Model file for the job. Use its own axes, mm. Face numbers are marked on the shaded views. A direction names the side the tool comes from. Coordinates: 2 decimals unless noted, no trailing zeros. Write each loop counter-clockwise with the first axis right and the second up, starting at its lowest first coordinate (ties: lowest second). Pieces come first, ordered by that corner, then holes. Notation, with made-up numbers: M 32.5,14.25 L 67.5,14.25 A6 ccw 67.5,22.25 Z; hole C -22.75,75 d6. An arc over 180 degrees is marked long. One line per question, with ' | ' between items. Start each with the question number.
(1) Two-plate mould, pull along X, no slides. Class the marked faces 3, 4 and 5: +X half, -X half, draft (parallel to the pull), parting line (faces both ways), or undercut.
(2) Tool access for the marked faces 1 and 2: list every direction of +Z, -Z, +X, -X, +Y, -Y with a clear straight run to the whole face (end or side of a thin tool).
(3) Flat gauge pins, fed straight in: pin 1 Ø2 at (x, y) = (-4, 3.5) entering from -Z; pin 2 Ø6.5 at (x, y) = (0, 0) entering from +Z; pin 3 Ø1.5 at (y, z) = (-3.5, 1.5) entering from +X. Where does each tip first touch, or does it go through?
(4) Wall check: probe 1 along Y at (x, z) = (0, 1.2); probe 2 along Z at (x, y) = (-6, -2); probe 3 along Z at (x, y) = (-2, 1.75). Give the ranges that are in metal, low to high.
(5) Cut at C-C (y = 0). Write the cut outline in (x, z).
(6) Cut at B-B (z = 1.2). Write the cut outline in (x, y), plus the area to 3 significant figures.
(7) Cut at A-A (x = 0). Write the cut outline in (y, z), plus the area to 3 significant figures.
from build123d import *

# Parameters (mm, degrees)
SKETCH_R        = 2.5
PAD_DEPTH       = 0.6
SKETCH002_R     = 9.5
PAD001_DEPTH    = 1
SKETCH003_R     = 9.5
SKETCH003_R_2   = 8
PAD002_DEPTH    = 1
SKETCH004_R     = 2.5
POCKET_DEPTH    = 1.601
CHAMFER_SIZE    = 0.4
CHAMFER001_SIZE = 0.2


with BuildPart() as part:
    # Sketch → Pad (new body)
    with BuildSketch(Plane.XY):
        with BuildLine():
            ThreePointArc((-2.5, 3.122499), (-3.518971, 1.901799), (-3.981855, 0.380567))
            Line((-5.478695, -0.483634), (-3.981855, 0.380567))
            ThreePointArc((-5.478695, -0.483634), (-4.659167, -2.922699), (-2.81991, -4.722087))
            Line((-1.232265, -3.80546), (-2.81991, -4.722087))
            ThreePointArc((-1.232265, -3.80546), (0.117848, -3.998264), (1.454262, -3.726275))
            Line((2.992718, -4.614503), (1.454262, -3.726275))
            ThreePointArc((2.992718, -4.614503), (4.763149, -2.749985), (5.492638, -0.284484))
            Line((3.954108, 0.604177), (5.492638, -0.284484))
            ThreePointArc((3.954108, 0.604177), (3.46401, 2.000159), (2.5, 3.122499))
            Line((2.5, 3.122499), (2.5, 4.898979))
            ThreePointArc((2.5, 4.898979), (0, 5.5), (-2.5, 4.898979))
            Line((-2.5, 3.122499), (-2.5, 4.898979))
        make_face()
        Circle(SKETCH_R, mode=Mode.SUBTRACT)
    extrude(amount=PAD_DEPTH)

    # Sketch002 (on Face15 of Pad) → Pad001 (join)
    with BuildSketch(Plane.XY.offset(0.6)):
        Circle(SKETCH002_R)
    extrude(amount=PAD001_DEPTH)

    # Sketch003 (on Face3 of Pad001) → Pad002 (join)
    with BuildSketch(Plane.XY.offset(1.6)):
        Circle(SKETCH003_R)
        Circle(SKETCH003_R_2, mode=Mode.SUBTRACT)
    extrude(amount=PAD002_DEPTH)

    # Sketch004 (on Face20 of Pad002) → Pocket (cut, through all)
    with BuildSketch(Plane.XY.offset(1.6)):
        Circle(SKETCH004_R)
    extrude(amount=-POCKET_DEPTH, mode=Mode.SUBTRACT)

    # Chamfer
    chamfer_edges = [part.edges().sort_by_distance(p)[0] for p in [
        (-8, 0, 2.6),
    ]]
    chamfer(chamfer_edges, length=CHAMFER_SIZE)

    # Chamfer001
    chamfer001_edges = [part.edges().sort_by_distance(p)[0] for p in [
        (4.723373, 0.159847, 0),
        (4.763149, -2.749985, 0),
        (0.117848, -3.998264, 0),
        (-2.026088, -4.263773, 0),
        (-4.659167, -2.922699, 0),
        (-4.730275, -0.051534, 0),
        (-3.518971, 1.901799, 0),
        (-2.5, 4.010739, 0),
        (0, 5.5, 0),
        (2.5, 4.010739, 0),
        (3.46401, 2.000159, 0),
    ]]
    chamfer(chamfer001_edges, length=CHAMFER001_SIZE)


solid = part.part
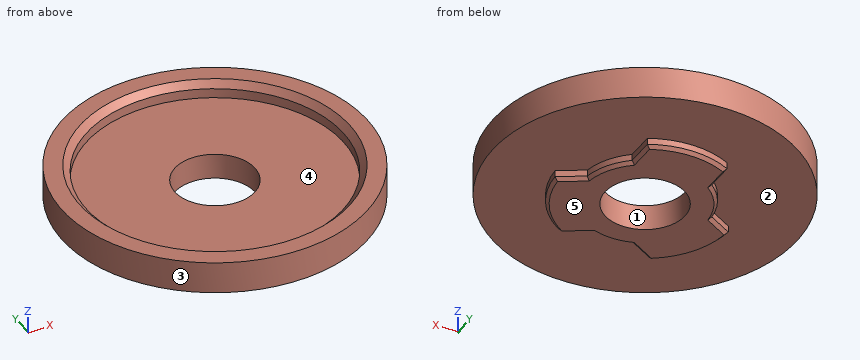
Filled in:
1) face 3: parting line | face 4: undercut | face 5: draft
2) face 1: +Z, -Z | face 2: -Z
3) pin 1: z = 0.6 | pin 2: z = 1.6 | pin 3: x = 9.09
4) probe 1: -9.5 to -2.5, 2.5 to 9.5 | probe 2: 0.6 to 1.6 | probe 3: 0 to 1.6
5) outline: M -9.5,0.6 L -4.64,0.6 L -4.64,0.2 L -4.24,0 L -2.5,0 L -2.5,1.6 L -8,1.6 L -8,2.2 L -8.4,2.6 L -9.5,2.6 Z; M 2.5,0 L 4.6,0 L 5,0.2 L 5,0.6 L 9.5,0.6 L 9.5,2.6 L 8.4,2.6 L 8,2.2 L 8,1.6 L 2.5,1.6 Z
6) outline: C 0,0 d19; hole C 0,0 d5 | area: 264 mm²
7) outline: M -9.5,0.6 L -4,0.6 L -4,0.2 L -3.8,0 L -2.5,0 L -2.5,1.6 L -8,1.6 L -8,2.2 L -8.4,2.6 L -9.5,2.6 Z; M 2.5,0 L 5.3,0 L 5.5,0.2 L 5.5,0.6 L 9.5,0.6 L 9.5,2.6 L 8.4,2.6 L 8,2.2 L 8,1.6 L 2.5,1.6 Z | area: 19.5 mm²
